```python
from build123d import *

# Parameters (mm, degrees)
OUTPUT_MASTER_SKETCH_R  = 25
BOSS_EXTRUDE1_DEPTH     = 9
SKETCH4_R               = 3.05
CUT_EXTRUDE1_DEPTH      = 4
SKETCH5_R               = 25.5
SKETCH5_R_2             = 25
BOSS_EXTRUDE2_DEPTH     = 0.5
SKETCH6_R               = 1.55
CUT_EXTRUDE2_DEPTH      = 38.16853508
SKETCH7_R               = 2.3
CUT_EXTRUDE3_DEPTH      = 3.1
CHAMFER1_SIZE           = 0.5
SKETCH8_R               = 7
CUT_EXTRUDE4_DEPTH      = 10
SKETCH9_R               = 7.55
CUT_EXTRUDE5_DEPTH      = 4
SKETCH10_R              = 2.1
M4_THRU_DEPTH           = 38.16853508
CHAMFER3_SIZE           = 0.5
M4_START                = -8
M4_HEXNUT_CUT_DEPTH     = 3.8
SKETCH12_W              = 7.1
SKETCH12_H              = 3.8
M4_HEXNUT_SLOT_DEPTH    = 55.701131961
M4_HEXNUT_PATTERN_COUNT = 6


with BuildPart() as part:
    # Output Master Sketch → Boss-Extrude1 (new body)
    with BuildSketch(Plane.XY):
        Circle(OUTPUT_MASTER_SKETCH_R)
    extrude(amount=BOSS_EXTRUDE1_DEPTH)

    # Sketch4 → Cut-Extrude1 (cut)
    with BuildSketch(Plane.XY):
        with Locations((21, 0)):
            Circle(SKETCH4_R)
        with Locations((10.5, -18.186533479)):
            Circle(SKETCH4_R)
        with Locations((-10.5, -18.186533479)):
            Circle(SKETCH4_R)
        with Locations((-21, 0)):
            Circle(SKETCH4_R)
        with Locations((-10.5, 18.186533479)):
            Circle(SKETCH4_R)
        with Locations((10.5, 18.186533479)):
            Circle(SKETCH4_R)
    extrude(amount=CUT_EXTRUDE1_DEPTH, mode=Mode.SUBTRACT)

    # Sketch5 → Boss-Extrude2 (add)
    with BuildSketch(Plane(origin=(0, 0, 0), x_dir=(-1, 0, 0), z_dir=(0, 0, -1))):
        Circle(SKETCH5_R)
        Circle(SKETCH5_R_2, mode=Mode.SUBTRACT)
    extrude(amount=-BOSS_EXTRUDE2_DEPTH)

    # Sketch6 → Cut-Extrude2 (cut, through all)
    with BuildSketch(Plane(origin=(0, 0, 0), x_dir=(-1, 0, 0), z_dir=(0, 0, -1))):
        with Locations((-21, 0)):
            Circle(SKETCH6_R)
        with Locations((-10.5, 18.186533479)):
            Circle(SKETCH6_R)
        with Locations((10.5, 18.186533479)):
            Circle(SKETCH6_R)
        with Locations((21, 0)):
            Circle(SKETCH6_R)
        with Locations((10.5, -18.186533479)):
            Circle(SKETCH6_R)
        with Locations((-10.5, -18.186533479)):
            Circle(SKETCH6_R)
    extrude(amount=-CUT_EXTRUDE2_DEPTH, mode=Mode.SUBTRACT)

    # Sketch7 → Cut-Extrude3 (cut)
    with BuildSketch(Plane.XY.offset(9)):
        with Locations((-21, 0)):
            Circle(SKETCH7_R)
        with Locations((-10.5, 18.186533479)):
            Circle(SKETCH7_R)
        with Locations((10.5, 18.186533479)):
            Circle(SKETCH7_R)
        with Locations((21, 0)):
            Circle(SKETCH7_R)
        with Locations((10.5, -18.186533479)):
            Circle(SKETCH7_R)
        with Locations((-10.5, -18.186533479)):
            Circle(SKETCH7_R)
    extrude(amount=-CUT_EXTRUDE3_DEPTH, mode=Mode.SUBTRACT)

    # Chamfer1
    chamfer1_edges = [part.edges().sort_by_distance(p)[0] for p in [
        (-25, 0, 9),
    ]]
    chamfer(chamfer1_edges, length=CHAMFER1_SIZE)

    # Sketch8 → Cut-Extrude4 (cut)
    with BuildSketch(Plane(origin=(0, 0, 0), x_dir=(-1, 0, 0), z_dir=(0, 0, -1))):
        Circle(SKETCH8_R)
    extrude(amount=-CUT_EXTRUDE4_DEPTH, mode=Mode.SUBTRACT)

    # Sketch9 → Cut-Extrude5 (cut)
    with BuildSketch(Plane(origin=(0, 0, 0), x_dir=(-1, 0, 0), z_dir=(0, 0, -1))):
        Circle(SKETCH9_R)
    extrude(amount=-CUT_EXTRUDE5_DEPTH, mode=Mode.SUBTRACT)

    # Sketch10 → M4 Thru (cut, through all)
    with BuildSketch(Plane.XY.offset(9)):
        with Locations((0, 20)):
            Circle(SKETCH10_R)
        with Locations((17.320508076, 10)):
            Circle(SKETCH10_R)
        with Locations((17.320508076, -10)):
            Circle(SKETCH10_R)
        with Locations((0, -20)):
            Circle(SKETCH10_R)
        with Locations((-17.320508076, -10)):
            Circle(SKETCH10_R)
        with Locations((-17.320508076, 10)):
            Circle(SKETCH10_R)
    extrude(amount=-M4_THRU_DEPTH, mode=Mode.SUBTRACT)

    # Chamfer3
    chamfer3_edges = [part.edges().sort_by_distance(p)[0] for p in [
        (7, 0, 9),
    ]]
    chamfer(chamfer3_edges, length=CHAMFER3_SIZE)

    # Sketch11 → M4 Hexnut Cut (cut)
    with BuildSketch(Plane.XY.offset(9).offset(M4_START)):
        Polygon((0, 24.099186911), (-3.55, 22.049593456), (-3.55, 17.950406544), (0, 15.900813089), (3.55, 17.950406544), (3.55, 22.049593456), align=None)
    m4_hexnut_cut = extrude(amount=M4_HEXNUT_CUT_DEPTH, mode=Mode.SUBTRACT)

    # Sketch12 → M4 Hexnut Slot (cut, through all)
    with BuildSketch(Plane(origin=(0, 22.049593456, 0), x_dir=(1, 0, 0), z_dir=(0, 1, 0))):
        with Locations((0, -2.9)):
            Rectangle(SKETCH12_W, SKETCH12_H)
    m4_hexnut_slot = extrude(amount=M4_HEXNUT_SLOT_DEPTH, mode=Mode.SUBTRACT)

    # M4 Hexnut Pattern: M4 Hexnut Cut, M4 Hexnut Slot ×6 about axis
    m4_hexnut_pattern_axis = Axis((0, 0, 0), (0, 0, 1))
    add([m4_hexnut_cut.rotate(m4_hexnut_pattern_axis, i * 360 / M4_HEXNUT_PATTERN_COUNT) for i in range(1, M4_HEXNUT_PATTERN_COUNT)], mode=Mode.SUBTRACT)
    add([m4_hexnut_slot.rotate(m4_hexnut_pattern_axis, i * 360 / M4_HEXNUT_PATTERN_COUNT) for i in range(1, M4_HEXNUT_PATTERN_COUNT)], mode=Mode.SUBTRACT)


solid = part.part
```
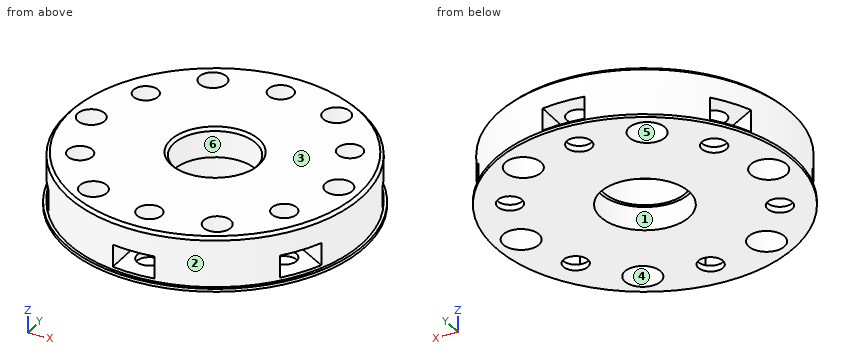
The listing builds one solid part. Answer for the finished solid, in the listing's coordinates (mm). Face numbers are marked on the shaded views. A direction names the side the tool comes from. Coordinates: 2 decimals unless noted, no trailing zeros.
Q1. Section A-A, the plane y = 0 is taken. Give the number of separate pieces and of enclosed holes in the cut face, then the cut area to 4 significant figures.
Returned:
separate pieces: 4
enclosed holes: 0
area: 230.5 mm2
Q2. The mould has two halves that part along Y. Classify the marked faces 1, 2, 3 and 4: released by +Y, released by -Y, zero draft, split by the parting line, or undercut.
Returned:
face 1: undercut
face 2: split by the parting line
face 3: zero draft
face 4: undercut
Q3. Given P1, Ø1.5, axis at y = 20, z = 7, coming from the +X side; P2, Ø3.5, axis at x = -10.5, y = -18.19, coming from the -Z side; P3, Ø3, axis at x = 21, y = 0, coming from the -Z side; P4, Ø4, axis at x = -10.5, y = 18.19, coming from the +Z side, each flat-ended and moving along its own axis, determine where each tip first touches the part or whether it passes through.
Returned:
P1: stops at x = 15.95
P2: stops at z = 4
P3: passes through
P4: stops at z = 5.9
Q4. Which of the six approach directions +Z, -Z, +X, -X, +Y, -Y give full straight-line access (tool end or side, diameter ignored) to the marked faces 5 and 6?
Returned:
face 5: -Z
face 6: +Z, -Z
Q5. Find the intervals of material crossed by line 1 along Z through (x, y) = (-21, 9.5); line 2 along Y through (x, z) = (0, 0.75); line 3 along X through (y, z) = (-9, 2.25), in increasing order.
Returned:
line 1: z = 0 to 1, 4.8 to 9
line 2: y = -25 to -22.1, -17.9 to -7.55, 7.55 to 17.9, 22.1 to 25
line 3: x = -23.32 to -22.69, -13.77 to 13.77, 22.69 to 23.32
